Design review of the part built by this model. Coordinates are the model's own, in mm. Coordinates: 2 decimals unless noted, no trailing zeros. Loops run counter-clockwise (first coordinate to the right, second up) from the corner with the lowest first, then second, coordinate; pieces in that order, holes last. Notation, with made-up numbers: (35.25, -36.5) -> (78.25, -36.5) arc R9 ccw to (78.25, -25.5) -> close; hole circle Ø9 at (50, 18). An arc over 180 degrees is marked (long way). Use a Markdown table: item, result. Add a question column.
Q1. Take a section at A-A on y = -4. Write out the cut boundary in (x, z).
Q2. Take a section at B-B on x = -1. Write out the cut boundary in (y, z).
Q3. Take a section at C-C on z = 1.4. Count the separate pieces of the cut face and the enclosed holes in it, plus the area to 3 significant figures.
Q4. For probe 1 along Y at (x, z) = (5, 1.45); probe 2 along Y at (x, z) = (-5, 2.05); probe 3 along X at (y, z) = (-24.45, 2.2), list the stretches that pass through material, from the lowest coordinate up.
Q5. Take a section at D-D on x = -5. Write out the cut boundary in (y, z), plus the area to 3 significant figures.
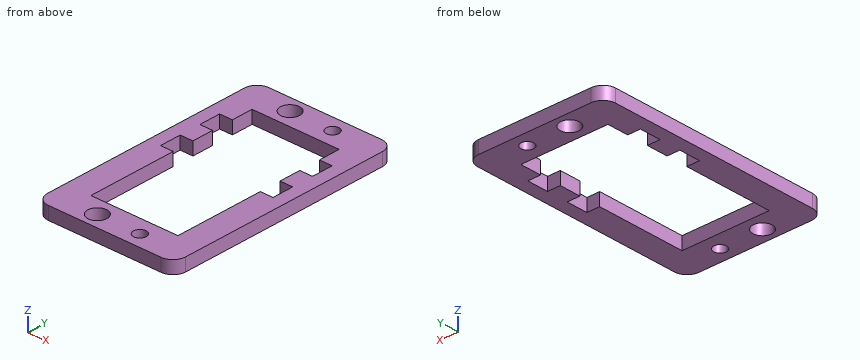
from build123d import *

# Parameters (mm, degrees)
SKETCH1_R           = 2.25
SKETCH1_R_2         = 1.5
BOSS_EXTRUDE1_DEPTH = 3


with BuildPart() as part:
    # Sketch1 → Boss-Extrude1 (new body)
    with BuildSketch(Plane.XY):
        with BuildLine():
            Line((-13.25, 27.95), (13.25, 27.95))
            ThreePointArc((13.25, 27.95), (15.371320344, 27.071320344), (16.25, 24.95))
            Line((16.25, 24.95), (16.25, -24.95))
            ThreePointArc((16.25, -24.95), (15.371320344, -27.071320344), (13.25, -27.95))
            Line((13.25, -27.95), (-13.25, -27.95))
            ThreePointArc((-13.25, -27.95), (-15.371320344, -27.071320344), (-16.25, -24.95))
            Line((-16.25, -24.95), (-16.25, 24.95))
            ThreePointArc((-16.25, 24.95), (-15.371320344, 27.071320344), (-13.25, 27.95))
        make_face()
        with Locations((-5, 24.45)):
            Circle(SKETCH1_R, mode=Mode.SUBTRACT)
        with Locations((5, 24.45)):
            Circle(SKETCH1_R_2, mode=Mode.SUBTRACT)
        with Locations(Location((5, -24.45, 0), (0, 0, 180))):
            Circle(SKETCH1_R_2, mode=Mode.SUBTRACT)
        with Locations(Location((-5, -24.45, 0), (0, 0, 180))):
            Circle(SKETCH1_R, mode=Mode.SUBTRACT)
        Polygon((-10.25, 20.45), (10.25, 20.45), (10.25, 15.45), (13.25, 15.45), (13.25, 10.45), (10.25, 10.45), (10.25, 5.45), (13.25, 5.45), (13.25, 0.45), (10.25, 0.45), (10.25, -20.45), (-10.25, -20.45), (-10.25, 0.45), (-13.25, 0.45), (-13.25, 5.45), (-10.25, 5.45), (-10.25, 10.45), (-13.25, 10.45), (-13.25, 15.45), (-10.25, 15.45), align=None, mode=Mode.SUBTRACT)
    extrude(amount=BOSS_EXTRUDE1_DEPTH)


solid = part.part
Answer list:
| question | item | result |
|---|---|---|
| 1 | outline | (-16.25, 0) -> (-10.25, 0) -> (-10.25, 3) -> (-16.25, 3) -> close; (10.25, 0) -> (16.25, 0) -> (16.25, 3) -> (10.25, 3) -> close |
| 2 | outline | (-27.95, 0) -> (-20.45, 0) -> (-20.45, 3) -> (-27.95, 3) -> close; (20.45, 0) -> (27.95, 0) -> (27.95, 3) -> (20.45, 3) -> close |
| 3 | separate pieces | 1 |
| 3 | enclosed holes | 5 |
| 3 | area | 865 mm² |
| 4 | probe 1 | -27.95 to -25.95, -22.95 to -20.45, 20.45 to 22.95, 25.95 to 27.95 |
| 4 | probe 2 | -27.95 to -26.7, -22.2 to -20.45, 20.45 to 22.2, 26.7 to 27.95 |
| 4 | probe 3 | -16.25 to -7.25, -2.75 to 3.5, 6.5 to 16.25 |
| 5 | outline | (-27.95, 0) -> (-26.7, 0) -> (-26.7, 3) -> (-27.95, 3) -> close; (-22.2, 0) -> (-20.45, 0) -> (-20.45, 3) -> (-22.2, 3) -> close; (20.45, 0) -> (22.2, 0) -> (22.2, 3) -> (20.45, 3) -> close; (26.7, 0) -> (27.95, 0) -> (27.95, 3) -> (26.7, 3) -> close |
| 5 | area | 18.0 mm² |
